from build123d import *

# Parameters (mm, degrees)
F0_W     = 42.3
F0_H     = 42.3
F1_DEPTH = 3
F2_D     = 4
F3_D     = 16


with BuildPart() as f1:
    # F0 (on Front) → F1 (new body)
    with BuildSketch(Plane.XZ):
        Rectangle(F0_W, F0_H)
    extrude(amount=F1_DEPTH)

    # F2 (through all)
    with Locations(Plane(origin=(0, 0, 0), x_dir=(1, 0, 0), z_dir=(0, 1, 0))):
        with Locations((-15.5, 15.5), (15.5, 15.5), (15.5, -15.5), (-15.5, -15.5)):
            Hole(F2_D / 2)

    # F3 (through all)
    with Locations(Plane(origin=(0, 0, 0), x_dir=(1, 0, 0), z_dir=(0, 1, 0))):
        with Locations((0, 0)):
            Hole(F3_D / 2)


solid = f1.part
Here's how the part is built. I have some questions about the finished solid (model axes, mm). Coordinates: 2 decimals unless noted, no trailing zeros. Loops run counter-clockwise (first coordinate to the right, second up) from the corner with the lowest first, then second, coordinate; pieces in that order, holes last.
1. Imagine slicing it at A-A, the plane x = 0. Please give me the cut outline in (y, z), and give its area (3 significant figures).
2. For P1, Ø3.5, axis at x = 15.5, z = -15.5, coming from the +Y side, with a flat end and sliding along its axis, tell me the tip position at first contact or that it passes through.
3. Imagine slicing it at B-B, the plane z = 0. Please give me the cut outline in (x, y).
4. Imagine slicing it at C-C, the plane y = -1.25. Please give me the cut outline in (x, z).
5. I need wall thicknesses on L1, parallel to X at y = -2, z = -15.5; L2, parallel to X at y = -0.5, z = 15. Which ranges of each line are inside material? Lowest first, please.
6. Imagine slicing it at D-D, the plane z = -15.5. Please give me the cut outline in (x, y).
7. If we mould it in two halves opening along Z, with no side actions, what happens to faces 1 (the cylindrical face through (15.76, -1.521, 13.517)), 2 (the flat face through (0, -1, -21.15)), 3 (the flat face through (21.15, -1, 0))? For each: pulls with the +Z half, pulls with the -Z half, needs draft (parallel to the pull), parting line crosses it, or undercut.
Taken from the geometry:
1. outline: (-3, -21.15) - (0, -21.15) - (0, -8) - (-3, -8) - close; (-3, 8) - (0, 8) - (0, 21.15) - (-3, 21.15) - close
1. area: 78.9 mm2
2. P1: passes through
3. outline: (-21.15, -3) - (-8, -3) - (-8, 0) - (-21.15, 0) - close; (8, -3) - (21.15, -3) - (21.15, 0) - (8, 0) - close
4. outline: (-21.15, -21.15) - (21.15, -21.15) - (21.15, 21.15) - (-21.15, 21.15) - close; hole circle Ø4 at (-15.5, -15.5); hole circle Ø4 at (-15.5, 15.5); hole circle Ø16 at (0, 0); hole circle Ø4 at (15.5, -15.5); hole circle Ø4 at (15.5, 15.5)
5. L1: x = -21.15 to -17.5, -13.5 to 13.5, 17.5 to 21.15
5. L2: x = -21.15 to -17.44, -13.56 to 13.56, 17.44 to 21.15
6. outline: (-21.15, -3) - (-17.5, -3) - (-17.5, 0) - (-21.15, 0) - close; (-13.5, -3) - (13.5, -3) - (13.5, 0) - (-13.5, 0) - close; (17.5, -3) - (21.15, -3) - (21.15, 0) - (17.5, 0) - close
7. face 1: undercut
7. face 2: pulls with the -Z half
7. face 3: needs draft
